from build123d import *

# Parameters (mm, degrees)
F2_R     = 25
F3_DEPTH = 100
F4_R     = 5
F5_DEPTH = 150.001


with BuildPart() as f1:
    # F0 (on Front) → F1 (revolve)
    with BuildSketch(Plane.XZ):
        Polygon((-31, 0), (0, 0), (0, 150), (-7, 150), (-7, 138), (-15, 138), (-15, 126), (-23, 126), (-23, 114), (-31, 114), align=None)
    revolve(axis=Axis((0, 0, 75), (0, 0, 1)))

    # F2 (on Top) → F3 (cut)
    with BuildSketch(Plane.XY):
        Circle(F2_R)
    extrude(amount=F3_DEPTH, mode=Mode.SUBTRACT)

    # F4 (on Top) → F5 (cut, through all)
    with BuildSketch(Plane.XY):
        Circle(F4_R)
    extrude(amount=F5_DEPTH, mode=Mode.SUBTRACT)


solid = f1.part
Could you check a few things on this model? Use its own coordinates, in mm. A direction names the side the tool comes from. Give positions to 0.01 mm unless a question says otherwise; leave off trailing zeros. Order: outer loops, then holes, each group sorted by start corner. A loop starts at its lowest first (then second) coordinate and runs counter-clockwise, first axis right, second up. Notation, with made-up numbers: (-8.75, -13.5) -> (7.25, -13.5) arc R22 ccw to (7.25, 20.5) -> close; hole circle Ø11 at (68, 2). An arc over 180 degrees is marked (long way). Return JSON: item names as keys, results as strings.
1. Imagine slicing it at A-A on y = 0. List the corners of the cut face in (x, z) for me, then the cut area to 3 significant figures.
Answer list:
{"outline": "(-31, 0) -> (-25, 0) -> (-25, 100) -> (-5, 100) -> (-5, 150) -> (-7, 150) -> (-7, 138) -> (-15, 138) -> (-15, 126) -> (-23, 126) -> (-23, 114) -> (-31, 114) -> close; (5, 100) -> (25, 100) -> (25, 0) -> (31, 0) -> (31, 114) -> (23, 114) -> (23, 126) -> (15, 126) -> (15, 138) -> (7, 138) -> (7, 150) -> (5, 150) -> close", "area": "2,650 mm2"}
2. I need wall thicknesses on line 1 (Y direction, x = 0, z = 38.5); line 2 (X direction, y = 0, z = 125). Which ranges of each line are inside material? Lowest first, please. Write a range as from..to.
Answer list:
{"line 1": "y = -31..-25, 25..31", "line 2": "x = -23..-5, 5..23"}
3. Thinking about a two-plate mould opening in Y: for faces 1 (the cylindrical face through (23.846, 7.509, 49.3)), 2 (the flat face through (-0.3, -5.2, 100)), 3 (the cylindrical face through (2.994, -22.804, 119.916)), 4 (the flat face through (3.1, 6.5, 138)), which applies, pulls with the +Y half, pulls with the -Y half, needs draft (parallel to the pull), parting line crosses it, or undercut?
Answer list:
{"face 1": "undercut", "face 2": "undercut", "face 3": "parting line crosses it", "face 4": "needs draft"}
4. On a 3-axis mill with a long thin cutter (end or side, diameter ignored), from which of +Z, -Z, +X, -X, +Y, -Y can I reach the whole of each face in a straight line? I mean faces 5 (the flat face through (-2, -5, 150)), 6 (the cylindrical face through (-6.466, 2.681, 143.916)). Say none if no direction works.
Answer list:
{"face 5": "+Z, +X, -X, +Y, -Y", "face 6": "+Z"}
5. Imagine slicing it at D-D on x = -10.5. List the corners of the cut face in (y, z) for me.
Answer list:
{"outline": "(-29.17, 0) -> (-22.69, 0) -> (-22.69, 100) -> (22.69, 100) -> (22.69, 0) -> (29.17, 0) -> (29.17, 114) -> (20.46, 114) -> (20.46, 126) -> (10.71, 126) -> (10.71, 138) -> (-10.71, 138) -> (-10.71, 126) -> (-20.46, 126) -> (-20.46, 114) -> (-29.17, 114) -> close"}
6. Imagine slicing it at C-C on z = 135. List the corners of the cut face in (x, y) for me.
Answer list:
{"outline": "circle Ø30 at (0, 0); hole circle Ø10 at (0, 0)"}
7. For pin 1 Ø5 at (y, z) = (17.5, 113) entering from +X; pin 2 Ø4 at (x, z) = (1, 40.5) entering from -Y; pin 3 Ø1 at (x, y) = (-10, -23) entering from +Z, each with a flat end and sliding along its axis, tell me the tip position at first contact or that it passes through.
Answer list:
{"pin 1": "stops at x = 27.13", "pin 2": "stops at y = -31", "pin 3": "stops at z = 114"}
